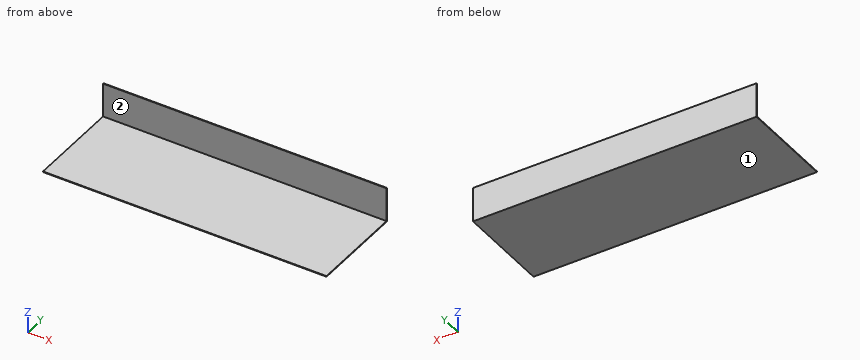
```python
from build123d import *

# Parameters (mm, degrees)
F0_W      = 2500
F0_H      = 840
F1_DEPTH  = 6
F2_W      = 2500
F2_H      = 6
F3_DEPTH  = 25
F3_FACE_W = 2500
F3_FACE_H = 6
F4_DEPTH  = 275


with BuildPart() as f1:
    # F0 (on Top) → F1 (new body)
    with BuildSketch(Plane.XY):
        with Locations((1151.201837, 401.51958)):
            Rectangle(F0_W, F0_H)
    extrude(amount=F1_DEPTH)

    # F2 (on face) → F3 (join)
    with BuildSketch(Plane.XY.offset(6)):
        with Locations((1151.201837, 818.51958)):
            Rectangle(F2_W, F2_H)
    extrude(amount=F3_DEPTH)

    # F3_face (on face) → F4 (join)
    with BuildSketch(Plane(origin=(1151.201837, 818.51958, 31), x_dir=(1, 0, 0), z_dir=(0, 0, 1))):
        Rectangle(F3_FACE_W, F3_FACE_H)
    extrude(amount=F4_DEPTH)


solid = f1.part
```
Source: CAD feature listing. Evaluate the final solid. Frame: model axes, mm. Face numbers are marked on the shaded views. A direction names the side the tool comes from. Round coordinates to 2 decimals unless told otherwise and drop trailing zeros. Loops run counter-clockwise (first coordinate to the right, second up) from the corner with the lowest first, then second, coordinate; pieces in that order, holes last. Notation, with made-up numbers: M 2,-28.5 L 26,-28.5 A28 ccw 26,-9.5 Z; hole C 78.25,43 d11. An arc over 180 degrees is marked long. Use a Markdown table: item, result. Add a question column.
1. Line query: line 1 (Z direction, x = 579, y = 268); line 2 (Y direction, x = 866.5, z = 244.5). Output: solid intervals per line, ascending.
2. Section query A-A on x = 1043. Return the cut outline in (y, z), then the cut area to 3 significant figures.
3. Section query C-C on y = 464. Return the cut outline in (x, z).
4. Contact query for flat-ended pins moving along their axis: P1, Ø6, axis at x = 191.5, z = 178, coming from the -Y side; P2, Ø12, axis at x = 1707.5, y = 716.5, coming from the +Z side. Output: stop coordinate, or through.
5. Section query B-B on z = 79.5. Return the cut outline in (x, y).
6. Reachability of the marked faces 1 and 2 from +Z, -Z, +X, -X, +Y, -Y: full face, straight path, thin tool, end or side. Return the list, or none.
Reported:
| question | item | result |
|---|---|---|
| 1 | line 1 | z = 0 to 6 |
| 1 | line 2 | y = 815.52 to 821.52 |
| 2 | outline | M -18.48,0 L 821.52,0 L 821.52,306 L 815.52,306 L 815.52,6 L -18.48,6 Z |
| 2 | area | 6,840 mm² |
| 3 | outline | M -98.8,0 L 2401.2,0 L 2401.2,6 L -98.8,6 Z |
| 4 | P1 | stops at y = 815.52 |
| 4 | P2 | stops at z = 6 |
| 5 | outline | M -98.8,815.52 L 2401.2,815.52 L 2401.2,821.52 L -98.8,821.52 Z |
| 6 | face 1 | -Z, +X, -X, +Y, -Y |
| 6 | face 2 | +Z, +X, -X, -Y |
